Model file for the job. Use its own axes, mm. Round coordinates to 2 decimals unless told otherwise and drop trailing zeros. One line per item, written item: value.
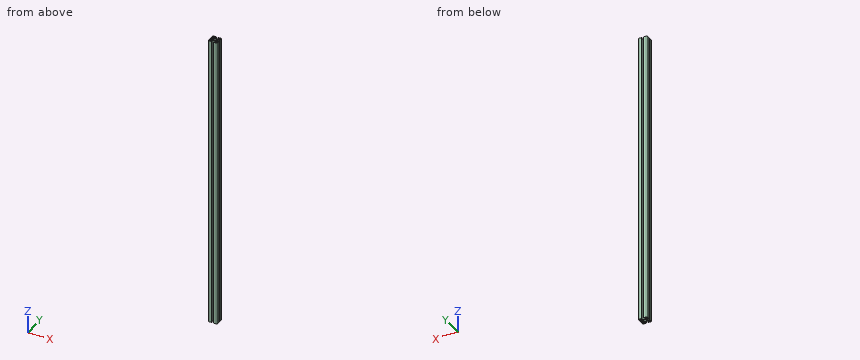
Autodesk Inventor part; units mm, degrees
ref_plane "side_4d_XY" through (-20, 0, -680) normal (-1, 0, 0) x (0, 1, 0)
ref_plane "side_4d_YZ" through (-20, 0, -680) normal (0, 1, 0) x (0, 0, -1)
ref_plane "side_4d_ZX" through (-20, 0, -680) normal (0, 0, -1) x (-1, 0, 0)
sketch "Skizze_1" plane through (0, 0, 0) normal (0, 0, 1) x (1, 0, 0)
  arc A0 (-20, -17) -> (-17, -20) centre (-17, -17) ccw
  line L0 (-17, -20) -> (-4.1, -20)
  line L1 (-4.1, -20) -> (-4.1, -17)
  line L2 (-4.1, -17) -> (-10.5, -17)
  line L3 (-10.5, -17) -> (-10.5, -13.6627)
  arc A1 (-10.0314, -12.5314) -> (-10.5, -13.6627) centre (-8.9002, -13.6627) ccw
  line L4 (-10.0314, -12.5314) -> (-7.4645, -9.9645)
  arc A2 (-3.9289, -8.5) -> (-7.4645, -9.9645) centre (-3.9289, -13.5) ccw
  line L5 (-3.9289, -8.5) -> (3.9289, -8.5)
  arc A3 (7.4645, -9.9645) -> (3.9289, -8.5) centre (3.9289, -13.5) ccw
  line L6 (7.4645, -9.9645) -> (10.0314, -12.5314)
  arc A4 (10.5, -13.6627) -> (10.0314, -12.5314) centre (8.9002, -13.6627) ccw
  line L7 (10.5, -13.6627) -> (10.5, -17)
  line L8 (10.5, -17) -> (4.1, -17)
  line L9 (4.1, -17) -> (4.1, -20)
  line L10 (4.1, -20) -> (17, -20)
  arc A5 (17, -20) -> (20, -17) centre (17, -17) ccw
  line L11 (20, -17) -> (20, -4.1)
  line L12 (20, -4.1) -> (17, -4.1)
  line L13 (17, -4.1) -> (17, -10.5)
  line L14 (17, -10.5) -> (13.6627, -10.5)
  arc A6 (12.5314, -10.0314) -> (13.6627, -10.5) centre (13.6627, -8.9002) ccw
  line L15 (12.5314, -10.0314) -> (9.9645, -7.4645)
  arc A7 (8.5, -3.9289) -> (9.9645, -7.4645) centre (13.5, -3.9289) ccw
  line L16 (8.5, -3.9289) -> (8.5, 3.9289)
  arc A8 (9.9645, 7.4645) -> (8.5, 3.9289) centre (13.5, 3.9289) ccw
  line L17 (9.9645, 7.4645) -> (12.5314, 10.0314)
  arc A9 (13.6627, 10.5) -> (12.5314, 10.0314) centre (13.6627, 8.9002) ccw
  line L18 (13.6627, 10.5) -> (17, 10.5)
  line L19 (17, 10.5) -> (17, 4.1)
  line L20 (17, 4.1) -> (20, 4.1)
  line L21 (20, 4.1) -> (20, 17)
  arc A10 (20, 17) -> (17, 20) centre (17, 17) ccw
  line L22 (17, 20) -> (4.1, 20)
  line L23 (4.1, 20) -> (4.1, 17)
  line L24 (4.1, 17) -> (10.5, 17)
  line L25 (10.5, 17) -> (10.5, 13.6627)
  arc A11 (10.0314, 12.5314) -> (10.5, 13.6627) centre (8.9002, 13.6627) ccw
  line L26 (10.0314, 12.5314) -> (7.4645, 9.9645)
  arc A12 (3.9289, 8.5) -> (7.4645, 9.9645) centre (3.9289, 13.5) ccw
  line L27 (3.9289, 8.5) -> (-3.9289, 8.5)
  arc A13 (-7.4645, 9.9645) -> (-3.9289, 8.5) centre (-3.9289, 13.5) ccw
  line L28 (-7.4645, 9.9645) -> (-10.0314, 12.5314)
  arc A14 (-10.5, 13.6627) -> (-10.0314, 12.5314) centre (-8.9002, 13.6627) ccw
  line L29 (-10.5, 13.6627) -> (-10.5, 17)
  line L30 (-10.5, 17) -> (-4.1, 17)
  line L31 (-4.1, 17) -> (-4.1, 20)
  line L32 (-4.1, 20) -> (-17, 20)
  arc A15 (-17, 20) -> (-20, 17) centre (-17, 17) ccw
  line L33 (-20, 17) -> (-20, 4.1)
  line L34 (-20, 4.1) -> (-17, 4.1)
  line L35 (-17, 4.1) -> (-17, 10.5)
  line L36 (-17, 10.5) -> (-13.6627, 10.5)
  arc A16 (-12.5314, 10.0314) -> (-13.6627, 10.5) centre (-13.6627, 8.9002) ccw
  line L37 (-12.5314, 10.0314) -> (-9.9645, 7.4645)
  arc A17 (-8.5, 3.9289) -> (-9.9645, 7.4645) centre (-13.5, 3.9289) ccw
  line L38 (-8.5, 3.9289) -> (-8.5, -3.9289)
  arc A18 (-9.9645, -7.4645) -> (-8.5, -3.9289) centre (-13.5, -3.9289) ccw
  line L39 (-9.9645, -7.4645) -> (-12.5314, -10.0314)
  arc A19 (-13.6627, -10.5) -> (-12.5314, -10.0314) centre (-13.6627, -8.9002) ccw
  line L40 (-13.6627, -10.5) -> (-17, -10.5)
  line L41 (-17, -10.5) -> (-17, -4.1)
  line L42 (-17, -4.1) -> (-20, -4.1)
  line L43 (-20, -4.1) -> (-20, -17)
  circle A20 centre (0, 0) radius 6
extrude "Extrusion1" add sketch "Skizze_1" against normal blind 1360
sketch "Sketch2" plane through (0, 0, 0) normal (0, 0, 1) x (1, 0, 0)
  point P0 (-15, -15)
hole "Drilling 1" at (-15, -15, 0) direction (0, 0, -1) diameter 5 depth 6000
sketch "Sketch3" plane through (0, 0, 0) normal (0, 0, 1) x (1, 0, 0)
  point P0 (15, -15)
hole "Drilling 2" at (15, -15, 0) direction (0, 0, -1) diameter 5 depth 6000
sketch "Sketch4" plane through (0, 0, 0) normal (0, 0, 1) x (1, 0, 0)
  point P0 (15, 15)
hole "Drilling 3" at (15, 15, 0) direction (0, 0, -1) diameter 5 depth 6000
sketch "Sketch5" plane through (0, 0, 0) normal (0, 0, 1) x (1, 0, 0)
  point P0 (-15, 15)
hole "Drilling 4" at (-15, 15, 0) direction (0, 0, -1) diameter 5 depth 6000
ref_plane "side_4d_XY" through (-20, 0, -680) normal (-1, 0, 0) x (0, 1, 0)
ref_plane "side_4d_YZ" through (-20, 0, -680) normal (0, 1, 0) x (0, 0, -1)
ref_plane "side_4d_ZX" through (-20, 0, -680) normal (0, 0, -1) x (-1, 0, 0)
ref_plane "side_1a_XY" through (0, 20, -680) normal (0, 1, 0) x (1, 0, 0)
ref_plane "side_1a_YZ" through (0, 20, -680) normal (1, 0, 0) x (0, 0, -1)
ref_plane "side_1a_ZX" through (0, 20, -680) normal (0, 0, -1) x (0, 1, 0)
ref_plane "side_2b_XY" through (20, 0, -680) normal (1, 0, 0) x (0, -1, 0)
ref_plane "side_2b_YZ" through (20, 0, -680) normal (0, -1, 0) x (0, 0, -1)
ref_plane "side_2b_ZX" through (20, 0, -680) normal (0, 0, -1) x (1, 0, 0)
ref_plane "side_3c_XY" through (0, -20, -680) normal (0, -1, 0) x (-1, 0, 0)
ref_plane "side_3c_YZ" through (0, -20, -680) normal (-1, 0, 0) x (0, 0, -1)
ref_plane "side_3c_ZX" through (0, -20, -680) normal (0, 0, -1) x (0, -1, 0)
ref_plane "end_XY" through (0, 0, -1360) normal (0, 0, -1) x (1, 0, 0)
ref_plane "end_YZ" through (0, 0, -1360) normal (1, 0, 0) x (0, -1, 0)
ref_plane "end_ZX" through (0, 0, -1360) normal (0, -1, 0) x (0, 0, -1)
ref_plane "start_XY" through (0, 0, 0) normal (0, 0, 1) x (1, 0, 0)
ref_plane "start_YZ" through (0, 0, 0) normal (1, 0, 0) x (0, 1, 0)
ref_plane "start_ZX" through (0, 0, 0) normal (0, 1, 0) x (0, 0, 1)
properties part number "MayTec 1.11.040040.43S_Profile 40x40, 4E, S_1360_Detail_(0;0,0,0)"
1. Wall check: probe 1 along Y at (x, z) = (-14, -982.5); probe 2 along X at (y, z) = (-15, -471.5). Give the ranges that are in metal, low to high. Write a range as [from, to].
Report:
probe 1: [-20, -17.29], [-12.71, -10.5], [10.5, 12.71], [17.29, 20]
probe 2: [-20, -17.5], [-12.5, -10.5], [10.5, 12.5], [17.5, 20]
2. Band-saw the part on A-A on z = -685.5. State how many separate pieces and enclosed holes the cut face has, plus the area to 3 significant figures.
Report:
separate pieces: 1
enclosed holes: 5
area: 674 mm²
3. Drop flat-ended pins along their axis: pin 1 (2.5 mm diameter, centred on x = 0.5, z = -1005, fed in from -Y); pin 2 (2.5 mm diameter, centred on y = 1.5, z = -614.5, fed in from +X); pin 3 (0.9 mm diameter, centred on y = 18, z = -735.5, fed in from +X). Give the stop position or say it passes through.
Report:
pin 1: y = -8.5
pin 2: x = 8.5
pin 3: x = 19.95
